Work out the finished part from the listing and answer in its coordinate system (mm). Face numbers are marked on the shaded views. Coordinates: 2 decimals unless noted, no trailing zeros. Loops run counter-clockwise (first coordinate to the right, second up) from the corner with the lowest first, then second, coordinate; pieces in that order, holes last. Notation, with made-up numbers: (-23, 65) - (-1, 65) arc R18 cw to (-1, 73) - close; hole circle Ø7 at (66, 34.5). An arc over 180 degrees is marked (long way). Write each question's results on one line, items separated by ' | '. Start each with the question number.
Item 1: Consider probe 1 along Y at (x, z) = (88.5, 10.5) (3 decimals); probe 2 along X at (y, z) = (4, 17.25); probe 3 along Z at (x, y) = (84, 2). Determine where each line is inside the solid, lowest interval first. Write a range as [from, to].
Item 2: Section A-A, the plane z = 10.5 is taken. Write down the section's boundary in (x, y) (3 decimals), plus the area to 3 significant figures.
Item 3: For a pull along Y with two mould halves and no side action, classify the marked faces 1, 2, 3 and 4 as +Y half, -Y half, draft (parallel to the pull), parting line (faces both ways), or undercut.
Item 4: Section B-B, the plane x = 117.5 is taken. Write down the section's boundary in (y, z) (3 decimals).
Item 5: Each of these flat-tipped pins is pushed along its axis until it touches: pin 1 Ø5.5 at (x, z) = (76, 10) entering from -Y; pin 2 Ø9.5 at (x, z) = (46.5, 12.5) entering from +Y; pin 3 Ø5 at (y, z) = (28, 14.5) entering from +X; pin 4 Ø1 at (x, y) = (83.5, 7) entering from +Z. Where does it stop, or does it pass through?
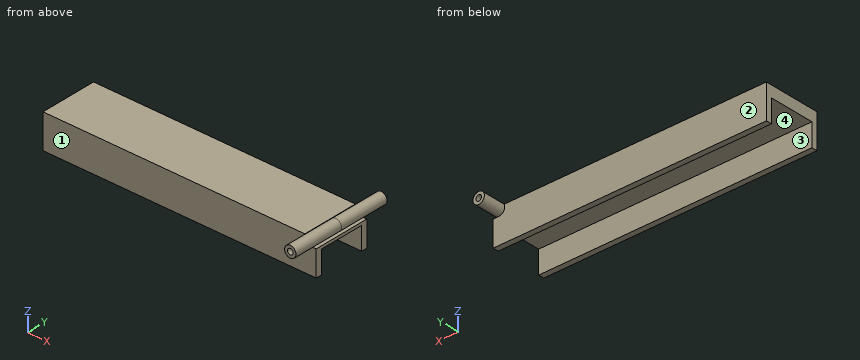
from build123d import *

# Parameters (mm, degrees)
F1_DEPTH      = 152.4
F2_W          = 152.4
F2_H          = 31.75
F3_DEPTH      = 3.175
F5_DEPTH      = 31.751
F7_R          = 3.175
F8_DEPTH      = 28.575
F8_DEPTH_BACK = 28.575
F9_R          = 1.5875
F10_DEPTH     = 57.151


with BuildPart() as f1:
    # F0 (on Right) → F1 (new body)
    with BuildSketch(Plane.YZ):
        Polygon((0, 15.875), (0, 0), (3.175, 0), (3.175, 12.7), (28.575, 12.7), (28.575, 0), (31.75, 0), (31.75, 15.875), align=None)
    extrude(amount=F1_DEPTH)

    # F2 (on face) → F3 (join)
    with BuildSketch(Plane.XY.offset(15.875)):
        with Locations((76.2, 15.875)):
            Rectangle(F2_W, F2_H)
    extrude(amount=F3_DEPTH)

    # F4 (on face) → F5 (cut, through all)
    with BuildSketch(Plane.XZ):
        with BuildLine():
            Line((146.05, 19.05), (146.05, 17.4625))
            ThreePointArc((146.05, 17.4625), (146.979936, 15.217436), (149.225, 14.2875))
            Line((149.225, 14.2875), (152.4, 14.2875))
            Line((152.4, 14.2875), (152.4, 17.4625))
            Line((152.4, 17.4625), (152.4, 19.05))
            Line((152.4, 19.05), (151.974631, 19.05))
            Line((151.974631, 19.05), (146.05, 19.05))
        make_face()
    extrude(amount=-F5_DEPTH, mode=Mode.SUBTRACT)

    # F7 (on offset) → F8 (join, two sides)
    with BuildSketch(Plane.XZ.offset(-15.875)) as f8_sk:
        with Locations((149.225, 17.4625)):
            Circle(F7_R)
    extrude(amount=F8_DEPTH)
    extrude(f8_sk.sketch, amount=-F8_DEPTH_BACK)

    # F9 (on face) → F10 (cut, through all)
    with BuildSketch(Plane.XZ.offset(12.7)):
        with Locations((149.225, 17.4625)):
            Circle(F9_R)
    extrude(amount=-F10_DEPTH, mode=Mode.SUBTRACT)


solid = f1.part
Answer key:
1) probe 1: y = [0, 3.175], [28.575, 31.75] | probe 2: x = [0, 147.65], [150.8, 152.39] | probe 3: z = [0, 19.05]
2) outline: (0, 0) - (152.4, 0) - (152.4, 3.175) - (0, 3.175) - close; (0, 28.575) - (152.4, 28.575) - (152.4, 31.75) - (0, 31.75) - close | area: 968 mm^2
3) face 1: -Y half | face 2: +Y half | face 3: undercut | face 4: undercut
4) outline: (0, 0) - (3.175, 0) - (3.175, 12.7) - (28.575, 12.7) - (28.575, 0) - (31.75, 0) - (31.75, 19.05) - (0, 19.05) - close
5) pin 1: stops at y = 0 | pin 2: stops at y = 31.75 | pin 3: stops at x = 152.4 | pin 4: stops at z = 19.05
